```python
from build123d import *

# Parameters (mm, degrees)
BOSS_EXTRUDE1_DEPTH = 2
BOSS_EXTRUDE2_DEPTH = 20
SKETCH3_R           = 12.5
CUT_EXTRUDE2_DEPTH  = 23
BOSS_EXTRUDE3_DEPTH = 1.5
SKETCH6_W           = 17.4
SKETCH6_H           = 16.7
SKETCH6_W_2         = 13.4
SKETCH6_H_2         = 12.7
BOSS_EXTRUDE4_DEPTH = 1
SKETCH7_W           = 11.6
SKETCH7_H           = 20
SKETCH7_R           = 3
BOSS_EXTRUDE5_DEPTH = 2
SKETCH8_W           = 4.8
SKETCH8_H           = 12
SKETCH8_H_2         = 20
BOSS_EXTRUDE6_DEPTH = 16.5
SKETCH9_R           = 0.5
CUT_EXTRUDE3_DEPTH  = 5
CUT_EXTRUDE4_DEPTH  = 2
SKETCH11_R          = 1.75
CUT_EXTRUDE5_DEPTH  = 2
CUT_EXTRUDE6_DEPTH  = 1


with BuildPart() as part:
    # Sketch1 → Boss-Extrude1 (new body)
    with BuildSketch(Plane(origin=(0, 0, 0), x_dir=(1, 0, 0), z_dir=(0, 1, 0))):
        with BuildLine():
            Line((-30, 25), (30, 25))
            ThreePointArc((30, 25), (40.606601718, 20.606601718), (45, 10))
            Line((45, 10), (45, -40))
            ThreePointArc((45, -40), (40.606601718, -50.606601718), (30, -55))
            Line((30, -55), (-30, -55))
            ThreePointArc((-30, -55), (-40.606601718, -50.606601718), (-45, -40))
            Line((-45, -40), (-45, 10))
            ThreePointArc((-45, 10), (-40.606601718, 20.606601718), (-30, 25))
        make_face()
    extrude(amount=BOSS_EXTRUDE1_DEPTH)

    # Sketch4 → Boss-Extrude2 (add)
    with BuildSketch(Plane(origin=(0, 2, 0), x_dir=(1, 0, 0), z_dir=(0, 1, 0))):
        with BuildLine():
            Line((30, 25), (-30, 25))
            ThreePointArc((-30, 25), (-40.606601718, 20.606601718), (-45, 10))
            Line((-45, 10), (-45, -40))
            ThreePointArc((-45, -40), (-40.606601718, -50.606601718), (-30, -55))
            Line((-30, -55), (30, -55))
            ThreePointArc((30, -55), (40.606601718, -50.606601718), (45, -40))
            Line((45, -40), (45, 10))
            ThreePointArc((45, 10), (40.606601718, 20.606601718), (30, 25))
        make_face()
        with BuildLine():
            Line((30, 23), (-30, 23))
            ThreePointArc((-30, 23), (-39.192388155, 19.192388155), (-43, 10))
            Line((-43, 10), (-43, -40))
            ThreePointArc((-43, -40), (-39.192388155, -49.192388155), (-30, -53))
            Line((-30, -53), (30, -53))
            ThreePointArc((30, -53), (39.192388155, -49.192388155), (43, -40))
            Line((43, -40), (43, 10))
            ThreePointArc((43, 10), (39.192388155, 19.192388155), (30, 23))
        make_face(mode=Mode.SUBTRACT)
    extrude(amount=BOSS_EXTRUDE2_DEPTH)

    # Sketch3 → Cut-Extrude2 (cut, through all)
    with BuildSketch(Plane.XZ):
        Circle(SKETCH3_R)
    extrude(amount=-CUT_EXTRUDE2_DEPTH, mode=Mode.SUBTRACT)

    # Sketch5 → Boss-Extrude3 (add)
    with BuildSketch(Plane(origin=(0, 2, 0), x_dir=(1, 0, 0), z_dir=(0, 1, 0))):
        Polygon((-36.002943725, -53), (5.1, -53), (5.1, -31), (-37.7, -31), (-37.7, -51.302943725), align=None)
    extrude(amount=BOSS_EXTRUDE3_DEPTH)

    # Sketch6 → Boss-Extrude4 (add)
    with BuildSketch(Plane(origin=(0, 2, 0), x_dir=(1, 0, 0), z_dir=(0, 1, 0))):
        with Locations((30.2, 0)):
            Rectangle(SKETCH6_W, SKETCH6_H)
        with Locations((30.2, 0)):
            Rectangle(SKETCH6_W_2, SKETCH6_H_2, mode=Mode.SUBTRACT)
    extrude(amount=BOSS_EXTRUDE4_DEPTH)

    # Sketch7 → Boss-Extrude5 (add)
    with BuildSketch(Plane.XY.offset(-23)):
        with Locations((-24.14, 12)):
            Rectangle(SKETCH7_W, SKETCH7_H)
        with Locations((-24.14, 11.75)):
            Circle(SKETCH7_R, mode=Mode.SUBTRACT)
    extrude(amount=BOSS_EXTRUDE5_DEPTH)

    # Sketch8 → Boss-Extrude6 (add)
    with BuildSketch(Plane(origin=(0, 3.5, 0), x_dir=(1, 0, 0), z_dir=(0, 1, 0))):
        with Locations((-35.3, -37)):
            Rectangle(SKETCH8_W, SKETCH8_H)
        with Locations((2.7, -41)):
            Rectangle(SKETCH8_W, SKETCH8_H_2)
    extrude(amount=BOSS_EXTRUDE6_DEPTH)

    # Sketch9 → Cut-Extrude3 (cut)
    with BuildSketch(Plane(origin=(0, 0, 31), x_dir=(-1, 0, 0), z_dir=(0, 0, -1))):
        with Locations((-2.7, 15.75)):
            Circle(SKETCH9_R)
        with Locations((-2.7, 7.75)):
            Circle(SKETCH9_R)
        with Locations((35.3, 15.75)):
            Circle(SKETCH9_R)
        with Locations((35.3, 7.75)):
            Circle(SKETCH9_R)
    extrude(amount=-CUT_EXTRUDE3_DEPTH, mode=Mode.SUBTRACT)

    # Sketch10 → Cut-Extrude4 (cut)
    with BuildSketch(Plane.XY.offset(55)):
        with BuildLine():
            Line((16, 22), (26, 22))
            Line((26, 22), (26, 19))
            ThreePointArc((26, 19), (25.414213562, 17.585786438), (24, 17))
            Line((24, 17), (18, 17))
            ThreePointArc((18, 17), (16.585786438, 17.585786438), (16, 19))
            Line((16, 19), (16, 22))
        make_face()
    extrude(amount=-CUT_EXTRUDE4_DEPTH, mode=Mode.SUBTRACT)

    # Sketch11 → Cut-Extrude5 (cut)
    with BuildSketch(Plane(origin=(-43, 0, 0), x_dir=(0, 0, -1), z_dir=(1, 0, 0))):
        with Locations((-30, 18.5)):
            Circle(SKETCH11_R)
        with Locations((0, 18.5)):
            Circle(SKETCH11_R)
    cut_extrude5 = extrude(amount=-CUT_EXTRUDE5_DEPTH, mode=Mode.SUBTRACT)

    # Sketch12 → Cut-Extrude6 (cut)
    with BuildSketch(Plane.ZY.offset(45)):
        with BuildLine():
            Line((-4, 22), (4, 22))
            Line((4, 22), (4, 18))
            ThreePointArc((4, 18), (3.121320344, 15.878679656), (1, 15))
            Line((1, 15), (-1, 15))
            ThreePointArc((-1, 15), (-3.121320344, 15.878679656), (-4, 18))
            Line((-4, 18), (-4, 22))
        make_face()
        with BuildLine():
            Line((26, 22), (34, 22))
            Line((34, 22), (34, 18))
            ThreePointArc((34, 18), (33.121320344, 15.878679656), (31, 15))
            Line((31, 15), (29, 15))
            ThreePointArc((29, 15), (26.878679656, 15.878679656), (26, 18))
            Line((26, 18), (26, 22))
        make_face()
    cut_extrude6 = extrude(amount=-CUT_EXTRUDE6_DEPTH, mode=Mode.SUBTRACT)

    # Mirror1: Cut-Extrude5, Cut-Extrude6 across plane
    add(cut_extrude5.mirror(Plane(origin=(0, 0, 0), x_dir=(0, 0, 1), z_dir=(1, 0, 0))), mode=Mode.SUBTRACT)
    add(cut_extrude6.mirror(Plane(origin=(0, 0, 0), x_dir=(0, 0, 1), z_dir=(1, 0, 0))), mode=Mode.SUBTRACT)


solid = part.part
```
Can you work these out from the model? Positions are in its coordinate system, mm. A direction names the side the tool comes from. Round coordinates to 2 decimals unless told otherwise and drop trailing zeros. Loops run counter-clockwise (first coordinate to the right, second up) from the corner with the lowest first, then second, coordinate; pieces in that order, holes last. Notation, with made-up numbers: (63, 44) -> (74, 44) arc R17 cw to (74, 69) -> close; hole circle Ø8 at (61, 47.25). An arc over 180 degrees is marked (long way). Answer in a Markdown table with one row per item.
Item 1: Suppose I cut it at C-C, the plane x = 6.5. List the corners of the cut face in (y, z) for me, plus the area to 3 significant figures.
Answer block:
| item | result |
|---|---|
| outline | (0, -25) -> (22, -25) -> (22, -23) -> (2, -23) -> (2, -10.68) -> (0, -10.68) -> close; (0, 10.68) -> (2, 10.68) -> (2, 53) -> (22, 53) -> (22, 55) -> (0, 55) -> close |
| area | 197 mm² |
Item 2: Suppose I cut it at D-D, the plane z = 30. List the corners of the cut face in (x, y) for me.
Answer block:
| item | result |
|---|---|
| outline | (-45, 0) -> (45, 0) -> (45, 15) -> (44, 15) -> (44, 16.75) -> (43, 16.75) -> (43, 2) -> (-43, 2) -> (-43, 16.75) -> (-44, 16.75) -> (-44, 15) -> (-45, 15) -> close; (-44, 20.25) -> (-43, 20.25) -> (-43, 22) -> (-44, 22) -> close; (43, 20.25) -> (44, 20.25) -> (44, 22) -> (43, 22) -> close |
Item 3: On a 3-axis mill with a long thin cutter (end or side, diameter ignored), from which of +Z, -Z, +X, -X, +Y, -Y can I reach the whole of each face in a straight line? I mean faces 5 (the cylindrical face through (-21.37, 10.6, -22.01)), 6 (the flat face through (21, 17, 54)), 7 (the cylindrical face through (-43.49, 19.68, 31.29)), 8 (the cylindrical face through (39.091, 11.86, 49.293)). Say none if no direction works.
Answer block:
| item | result |
|---|---|
| face 5 | none |
| face 6 | +Z, +Y |
| face 7 | -X |
| face 8 | +Y |
Item 4: Will these pins go through, and if not, where does the flat tip stop? P1, Ø3.5, axis at y = 18.5, z = -1, coming from the +X side; P2, Ø5.5, axis at x = -35.5, z = 38.5, coming from the +Y side; P3, Ø1, axis at y = 11.5, z = 46.5, coming from the -X side.
Answer block:
| item | result |
|---|---|
| P1 | x = 44 |
| P2 | y = 20 |
| P3 | x = -43.75 |
Item 5: If I drill on probe 1 along X at (y, z) = (4.5, 39.5); probe 2 along Z at (x, y) = (-19.5, 14); probe 3 along Z at (x, y) = (13.5, 6.75), over which ranges is the centre line in solid material (lowest first)?
Answer block:
| item | result |
|---|---|
| probe 1 | -45 to -43, -37.7 to -32.9, 0.3 to 5.1, 43 to 45 |
| probe 2 | -25 to -21, 53 to 55 |
| probe 3 | -25 to -23, 53 to 55 |
Item 6: We'd pull the mould along X, two halves only. Please class faces 1 (the cylindrical face through (-40.49, 10.85, -20.72)), 2 (the cylindrical face through (-43.493, 20.235, 0.228)), 3 (the flat face through (3, 20, 41)), 4 (the cylindrical face through (16.6, 17.57, 54.01)): released by +X, released by -X, zero draft, split by the parting line, or undercut.
Answer block:
| item | result |
|---|---|
| face 1 | released by -X |
| face 2 | zero draft |
| face 3 | undercut |
| face 4 | undercut |
Item 7: Suppose I cut it at A-A, the plane y = 11.75. Give the number of separate pieces and of enclosed holes in the cut face, plus the area to 3 significant figures.
Answer block:
| item | result |
|---|---|
| separate pieces | 3 |
| enclosed holes | 1 |
| area | 781 mm² |
